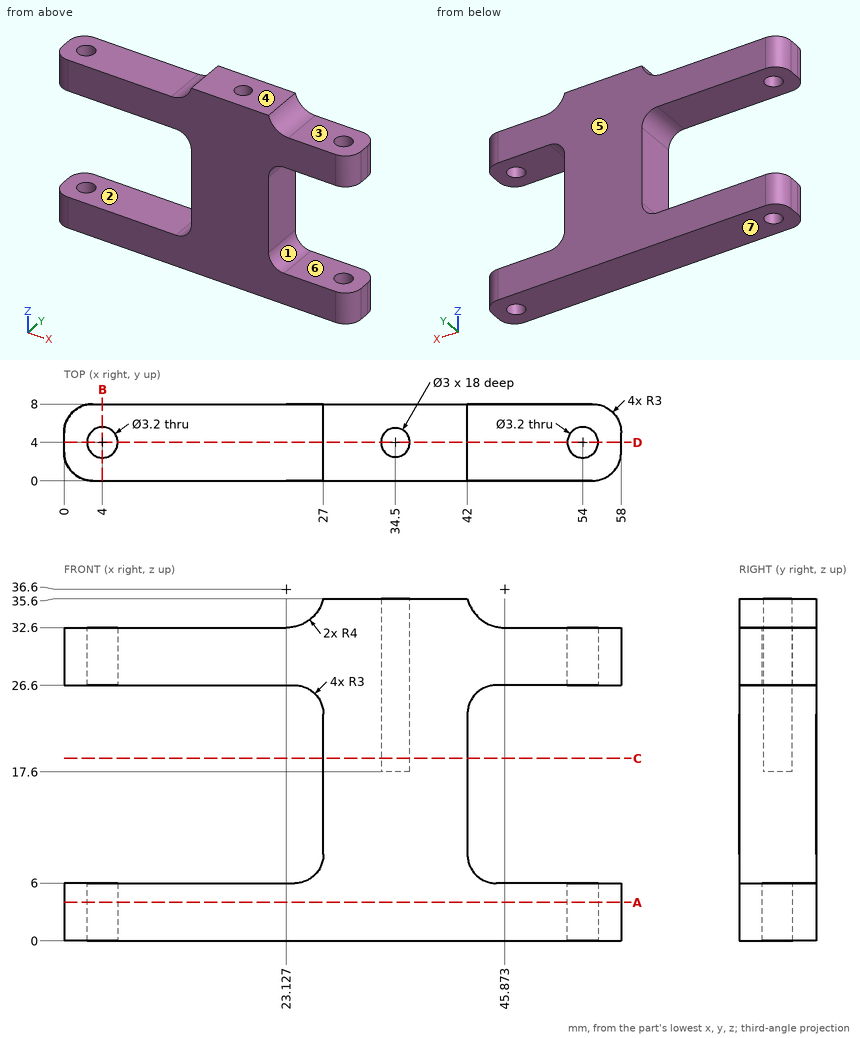
Input: dimensioned drawing with shaded views. Units: mm. Origin: part minimum x, y, z. A direction names the side the tool comes from. Coordinates: 2 decimals unless noted, no trailing zeros. Loops run counter-clockwise (first coordinate to the right, second up) from the corner with the lowest first, then second, coordinate; pieces in that order, holes last. Notation, with made-up numbers: M 40.5,-12.75 L 80.5,-12.75 A18 ccw 80.5,-3.75 Z; hole C -37.75,24 d5. An arc over 180 degrees is marked long. One line per item, written item: value.
(1) Section B-B (x = 4). Output: boundary loops of the cut face in (y, z).
Filled in:
outline: M 0,0 L 2.4,0 L 2.4,6 L 0,6 Z; M 0,26.6 L 2.4,26.6 L 2.4,32.6 L 0,32.6 Z; M 5.6,0 L 8,0 L 8,6 L 5.6,6 Z; M 5.6,26.6 L 8,26.6 L 8,32.6 L 5.6,32.6 Z
(2) Pin query (flat end, axial travel): pin 1 (2 mm diameter, centred on y = 5, z = 26, fed in from +X); pin 2 (4 mm diameter, centred on y = 5.5, z = 16.5, fed in from -X); pin 3 (2.5 mm diameter, centred on x = 12, y = 5.5, fed in from +Z); pin 4 (1 mm diameter, centred on y = 1.5, z = 8.5, fed in from +X). Return the tip coordinate at first contact, or that it passes through.
Filled in:
pin 1: x = 58
pin 2: x = 27
pin 3: z = 32.6
pin 4: x = 42.17
(3) Section A-A (z = 4). Output: boundary loops of the cut face in (x, y).
Filled in:
outline: M 0,3 A3 ccw 3,0 L 55,0 A3 ccw 58,3 L 58,5 A3 ccw 55,8 L 3,8 A3 ccw 0,5 Z; hole C 4,4 d3.2; hole C 54,4 d3.2
(4) Pull-direction query (Z, two-part tool) for the marked faces 4, 5, 6 and 7; classes: +Z half, -Z half, draft (parallel to the pull), parting line (faces both ways), or undercut.
Filled in:
face 4: +Z half
face 5: draft
face 6: undercut
face 7: -Z half
(5) Section C-C (z = 19). Output: boundary loops of the cut face in (x, y).
Filled in:
outline: M 27,0 L 42,0 L 42,8 L 27,8 Z; hole C 34.5,4 d3
(6) Section D-D (y = 4). Give the number of separate pieces and of enclosed holes in the cut face, and give its area (3 significant figures).
Filled in:
separate pieces: 5
enclosed holes: 0
area: 933 mm^2
(7) Reachability of the marked faces 1, 2 and 3 from +Z, -Z, +X, -X, +Y, -Y: full face, straight path, thin tool, end or side. Return the list, or none.
Filled in:
face 1: +X, +Y, -Y
face 2: -X, +Y, -Y
face 3: +Z, +X, +Y, -Y
(8) Line query: line 1 along Z through (x, y) = (11.5, 2.25); line 2 along Y through (x, z) = (54, 2.3); line 3 along Y through (x, z) = (34.5, 31). Output: solid intervals per line, ascending. Write a range as from..to.
Filled in:
line 1: 0..6, 26.6..32.6
line 2: 0..2.4, 5.6..8
line 3: 0..2.5, 5.5..8
